from build123d import *

# Parameters (mm, degrees)
SKETCH1_W           = 388
SKETCH1_H           = 289
SKETCH1_R           = 2
BOSS_EXTRUDE1_DEPTH = 1
SKETCH3_W           = 12
SKETCH3_H           = 120
BOSS_EXTRUDE2_DEPTH = 1
FILLET1_R           = 6


with BuildPart() as part:
    # Sketch1 → Boss-Extrude1 (new body)
    with BuildSketch(Plane.XY):
        Rectangle(SKETCH1_W, SKETCH1_H)
        with Locations((-182.759742869, 100.000000002)):
            Circle(SKETCH1_R, mode=Mode.SUBTRACT)
        with Locations((-182.759742868, 80.000000002)):
            Circle(SKETCH1_R, mode=Mode.SUBTRACT)
        with Locations((-182.759742869, -100)):
            Circle(SKETCH1_R, mode=Mode.SUBTRACT)
        with Locations((-182.759742869, -80)):
            Circle(SKETCH1_R, mode=Mode.SUBTRACT)
    extrude(amount=BOSS_EXTRUDE1_DEPTH)

    # Sketch3 → Boss-Extrude2 (add)
    with BuildSketch(Plane.XY.offset(1)):
        with Locations((200, 0)):
            Rectangle(SKETCH3_W, SKETCH3_H)
    extrude(amount=-BOSS_EXTRUDE2_DEPTH)

    # Fillet1
    fillet1_edges = [part.edges().sort_by_distance(p)[0] for p in [
        (194, -60, 0.5),
        (194, 60, 0.5),
    ]]
    fillet(fillet1_edges, radius=FILLET1_R)
    fillet1_2_edges = [part.edges().sort_by_distance(p)[0] for p in [
        (206, -60, 0.5),
        (206, 60, 0.5),
    ]]
    fillet(fillet1_2_edges, radius=FILLET1_R - 0.0001)  # a hair under: the kernel refuses the full size


solid = part.part
Can you work these out from the model? Positions are in its coordinate system, mm. Coordinates: 2 decimals unless noted, no trailing zeros. Write each loop counter-clockwise with the first axis right and the second up, starting at its lowest first coordinate (ties: lowest second). Pieces come first, ordered by that corner, then holes. Notation, with made-up numbers: (40.5, 51.25) -> (78.5, 51.25) arc R12 cw to (78.5, 73.25) -> close; hole circle Ø11 at (54, 87.25). An arc over 180 degrees is marked (long way). Write item = value, one per line.
(1) If I drill on probe 1 along X at (y, z) = (-66.5, 0.85), over which ranges is the centre line in solid material (lowest first)?
Verdict:
probe_1 = -194 to 194
(2) For pin 1 (0.5 mm diameter, centred on y = 96.5, z = 0.5, fed in from +X), with a flat end and sliding along its axis, tell me the tip position at first contact or that it passes through.
Verdict:
pin_1 = 194
(3) Imagine slicing it at A-A (z = 0.4). State how many separate pieces and enclosed holes the cut face has, and give its area (3 significant figures).
Verdict:
separate_pieces = 1
enclosed_holes = 4
area = 114,000 mm^2
(4) Imagine slicing it at B-B (y = -118). Please give me the cut outline in (x, z).
Verdict:
outline = (-194, 0) -> (194, 0) -> (194, 1) -> (-194, 1) -> close
